Model file for the job. Use its own axes, mm. Give positions to 0.01 mm unless a question says otherwise; leave off trailing zeros. Order: outer loops, then holes, each group sorted by start corner. A loop starts at its lowest first (then second) coordinate and runs counter-clockwise, first axis right, second up. Notation, with made-up numbers: (86.5, 10) - (116.5, 10) arc R21 cw to (116.5, 17) - close; hole circle Ø8 at (44, 5). An arc over 180 degrees is marked (long way). Return JSON: item names as keys, results as strings. Group by question number.
from build123d import *

# Parameters (mm, degrees)
F0_W     = 1119.75
F0_H     = 685.75
F1_DEPTH = 15
F3_DEPTH = 5
F4_R     = 3.5
F5_DEPTH = 10
F7_DEPTH = 15


with BuildPart() as f1:
    # F0 (on Top) → F1 (new body)
    with BuildSketch(Plane.XY):
        Rectangle(F0_W, F0_H)
    extrude(amount=F1_DEPTH)

    # F2 (on face) → F3 (cut)
    with BuildSketch(Plane.XY.offset(15)):
        with BuildLine():
            Line((0, 269), (0, 275))
            Line((0, 275), (-458.5, 275))
            Line((-458.5, 275), (-458.5, 284.5))
            ThreePointArc((-458.5, 284.5), (-459.37868, 286.62132), (-461.5, 287.5))
            Line((-461.5, 287.5), (-486.5, 287.5))
            ThreePointArc((-486.5, 287.5), (-488.62132, 286.62132), (-489.5, 284.5))
            Line((-489.5, 284.5), (-489.5, 259.5))
            ThreePointArc((-489.5, 259.5), (-488.62132, 257.37868), (-486.5, 256.5))
            Line((-486.5, 256.5), (-477, 256.5))
            Line((-477, 256.5), (-477, 0))
            Line((-477, 0), (-471, 0))
            Line((-471, 0), (-471, 256.5))
            Line((-471, 256.5), (-461.5, 256.5))
            ThreePointArc((-461.5, 256.5), (-459.37868, 257.37868), (-458.5, 259.5))
            Line((-458.5, 259.5), (-458.5, 269))
            Line((-458.5, 269), (0, 269))
        make_face()
        with BuildLine():
            Line((458.5, 275), (0, 275))
            Line((0, 275), (0, 269))
            Line((0, 269), (458.5, 269))
            Line((458.5, 269), (458.5, 259.5))
            ThreePointArc((458.5, 259.5), (459.37868, 257.37868), (461.5, 256.5))
            Line((461.5, 256.5), (471, 256.5))
            Line((471, 256.5), (471, 0))
            Line((471, 0), (471, -256.5))
            Line((471, -256.5), (461.5, -256.5))
            ThreePointArc((461.5, -256.5), (459.37868, -257.37868), (458.5, -259.5))
            Line((458.5, -259.5), (458.5, -269))
            Line((458.5, -269), (0, -269))
            Line((0, -269), (-458.5, -269))
            Line((-458.5, -269), (-458.5, -259.5))
            ThreePointArc((-458.5, -259.5), (-459.37868, -257.37868), (-461.5, -256.5))
            Line((-461.5, -256.5), (-471, -256.5))
            Line((-471, -256.5), (-471, 0))
            Line((-471, 0), (-477, 0))
            Line((-477, 0), (-477, -256.5))
            Line((-477, -256.5), (-486.5, -256.5))
            ThreePointArc((-486.5, -256.5), (-488.62132, -257.37868), (-489.5, -259.5))
            Line((-489.5, -259.5), (-489.5, -284.5))
            ThreePointArc((-489.5, -284.5), (-488.62132, -286.62132), (-486.5, -287.5))
            Line((-486.5, -287.5), (-461.5, -287.5))
            ThreePointArc((-461.5, -287.5), (-459.37868, -286.62132), (-458.5, -284.5))
            Line((-458.5, -284.5), (-458.5, -275))
            Line((-458.5, -275), (0, -275))
            Line((0, -275), (458.5, -275))
            Line((458.5, -275), (458.5, -284.5))
            ThreePointArc((458.5, -284.5), (459.37868, -286.62132), (461.5, -287.5))
            Line((461.5, -287.5), (486.5, -287.5))
            ThreePointArc((486.5, -287.5), (488.62132, -286.62132), (489.5, -284.5))
            Line((489.5, -284.5), (489.5, -259.5))
            ThreePointArc((489.5, -259.5), (488.62132, -257.37868), (486.5, -256.5))
            Line((486.5, -256.5), (477, -256.5))
            Line((477, -256.5), (477, 0))
            Line((477, 0), (477, 256.5))
            Line((477, 256.5), (486.5, 256.5))
            ThreePointArc((486.5, 256.5), (488.62132, 257.37868), (489.5, 259.5))
            Line((489.5, 259.5), (489.5, 284.5))
            ThreePointArc((489.5, 284.5), (488.62132, 286.62132), (486.5, 287.5))
            Line((486.5, 287.5), (461.5, 287.5))
            ThreePointArc((461.5, 287.5), (459.37868, 286.62132), (458.5, 284.5))
            Line((458.5, 284.5), (458.5, 275))
        make_face()
    extrude(amount=-F3_DEPTH, mode=Mode.SUBTRACT)

    # F4 (on face) → F5 (cut, through all)
    with BuildSketch(Plane.XY.offset(10)):
        with Locations((-474, 272)):
            Circle(F4_R)
        with Locations((474, -272)):
            Circle(F4_R)
        with Locations((-474, -272)):
            Circle(F4_R)
        with BuildLine():
            Line((484.5, 285.5), (463.5, 285.5))
            ThreePointArc((463.5, 285.5), (460.744077, 283.68528), (461.322307, 280.436592))
            Line((461.322307, 280.436592), (471.531947, 269.661471))
            ThreePointArc((471.531947, 269.661471), (472.656683, 268.876621), (474, 268.6))
            Line((474, 268.6), (484.5, 268.6))
            ThreePointArc((484.5, 268.6), (486.62132, 269.47868), (487.5, 271.6))
            Line((487.5, 271.6), (487.5, 282.5))
            ThreePointArc((487.5, 282.5), (486.62132, 284.62132), (484.5, 285.5))
        make_face()
    extrude(amount=-F5_DEPTH, mode=Mode.SUBTRACT)

    # F6 (on face) → F7 (cut, through all)
    with BuildSketch(Plane.XY.offset(15)):
        with BuildLine():
            Line((462.5, 262.5), (-462.5, 262.5))
            ThreePointArc((-462.5, 262.5), (-464.62132, 261.62132), (-465.5, 259.5))
            Line((-465.5, 259.5), (-465.5, -259.5))
            ThreePointArc((-465.5, -259.5), (-464.62132, -261.62132), (-462.5, -262.5))
            Line((-462.5, -262.5), (462.5, -262.5))
            ThreePointArc((462.5, -262.5), (464.62132, -261.62132), (465.5, -259.5))
            Line((465.5, -259.5), (465.5, 259.5))
            ThreePointArc((465.5, 259.5), (464.62132, 261.62132), (462.5, 262.5))
        make_face()
    extrude(amount=-F7_DEPTH, mode=Mode.SUBTRACT)


solid = f1.part
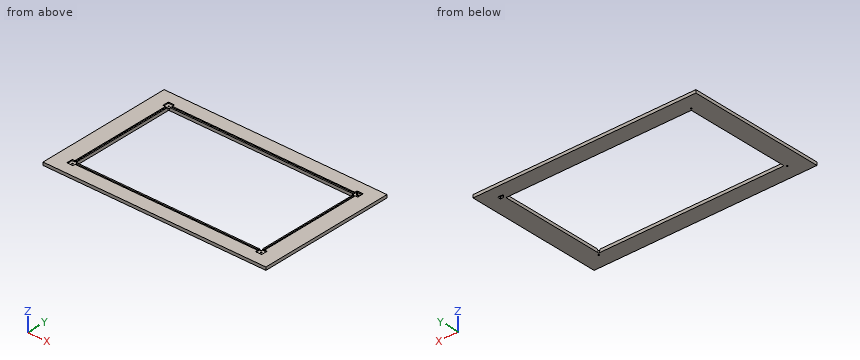
(1) Slice it at B-B (y = 207). Give the cut face in (x, z) (3 decimals), and give its area (3 significant figures).
(2) Drop a flat-ended pin along its axis: pin 1 Ø6.5 at (x, y) = (-474, -272) entering from -Z. Give the stop position or say it passes through.
(3) Slice it at A-A (x = -63). Give the cut face in (y, z) (3 decimals).
(4) Drill centre lines: L1, parallel to Y at x = 187, z = 12.25 (3 decimals); L2, parallel to X at y = -101.5, z = 10.5 (3 decimals); L3, parallel to Y at x = -474, z = 2.5 (3 decimals). Where is each one in solid material? Low to high.
Result set:
{
 "1": {"outline": "(-559.875, 0) - (-465.5, 0) - (-465.5, 15) - (-471, 15) - (-471, 10) - (-477, 10) - (-477, 15) - (-559.875, 15) - close; (465.5, 0) - (559.875, 0) - (559.875, 15) - (477, 15) - (477, 10) - (471, 10) - (471, 15) - (465.5, 15) - close", "area": "2,770 mm²"},
 "2": {"pin 1": "passes through"},
 "3": {"outline": "(-342.875, 0) - (-262.5, 0) - (-262.5, 15) - (-269, 15) - (-269, 10) - (-275, 10) - (-275, 15) - (-342.875, 15) - close; (262.5, 0) - (342.875, 0) - (342.875, 15) - (275, 15) - (275, 10) - (269, 10) - (269, 15) - (262.5, 15) - close"},
 "4": {"L1": "y = -342.875 to -275, -269 to -262.5, 262.5 to 269, 275 to 342.875", "L2": "x = -559.875 to -477, -471 to -465.5, 465.5 to 471, 477 to 559.875", "L3": "y = -342.875 to -275.5, -268.5 to 268.5, 275.5 to 342.875"}
}
